Read the model definition and answer for the solid it produces. Units are mm, in the model's axes. A direction names the side the tool comes from. Round coordinates to 2 decimals unless told otherwise and drop trailing zeros. Write each loop counter-clockwise with the first axis right and the second up, starting at its lowest first coordinate (ties: lowest second). Pieces come first, ordered by that corner, then holes. Notation, with made-up numbers: (13.5, 15) - (43.5, 15) arc R4 cw to (43.5, 22) - close; hole circle Ø2 at (45, 7). An arc over 180 degrees is marked (long way). One line per item, written item: value. Start each with the question number.
(1) A cutting plane is placed at D-D, the plane x = 17. Determine the outline of the cut face in (y, z).
(2) Find the intervals of material crossed by L1, parallel to Y at x = 10, z = 24; L2, parallel to X at y = 21.5, z = 22; L3, parallel to Y at x = -71, z = 9.5, in increasing order.
(3) Flat-ended cylindrical pins translate along their axes: pin 1 Ø12 at (x, z) = (35, 26.5) entering from +Y; pin 2 Ø1 at (y, z) = (-17, 23.5) entering from +X; pin 3 Ø10 at (x, z) = (-56, 17.5) entering from -Y. Find the tip coordinate at first contact, or state that the pin passes through.
(4) A cutting plane is placed at B-B, the plane z = 20. Determine the outline of the cut face in (x, y).
(5) For faces 3 (the face through (0, 22.5, 14)), 4 (the face through (-62.735, 49.663, 15.818)), determine the directions among +Z, -Z, +X, -X, +Y, -Y from which every point of the face is accessible in a straight line to the end or side of a thin tool.
(6) The mould has two halves that part along Y. Classify faces 1 (the face through (-1, 28, 0)), 2 (the face through (63.45, -46.67, 29.16)): +Y half, -Y half, draft (parallel to the pull), parting line (faces both ways), or undercut.
(7) A cutting plane is placed at C-C, the plane y = 38. State how many separate pieces and enclosed holes the cut face has, plus the area to 3 significant figures.
(8) A cutting plane is placed at A-A, the plane x = -50. Determine the outline of the cut face in (y, z), plus the area to 3 significant figures.
from build123d import *

# Parameters (mm, degrees)
F1_DEPTH = 3
F2_DEPTH = 30
F3_SIZE  = 1


with BuildPart() as f1:
    # F0 (on Top) → F1 (new body)
    with BuildSketch(Plane.XY):
        with BuildLine():
            Line((13.857919263, 32.5), (-13.857919263, 32.5))
            ThreePointArc((-13.857919263, 32.5), (-66.5376476243, 56.1564438266), (-80, 0))
            ThreePointArc((-80, 0), (-66.5376476243, -56.1564438266), (-13.857919263, -32.5))
            Line((-13.857919263, -32.5), (13.857919263, -32.5))
            ThreePointArc((13.857919263, -32.5), (66.5376476243, -56.1564438266), (80, 0))
            ThreePointArc((80, 0), (66.5376476243, 56.1564438266), (13.857919263, 32.5))
        make_face()
        with BuildLine():
            ThreePointArc((-69.843134833, 0), (-63.4726862442, 49.30460269), (-20.1043481422, 25))
            Line((-20.1043481422, 25), (20.1043481422, 25))
            ThreePointArc((20.1043481422, 25), (63.4726862442, 49.30460269), (69.843134833, 0))
            ThreePointArc((69.843134833, 0), (63.4726862442, -49.30460269), (20.1043481422, -25))
            Line((20.1043481422, -25), (-20.1043481422, -25))
            ThreePointArc((-20.1043481422, -25), (-63.4726862442, -49.30460269), (-69.843134833, 0))
        make_face(mode=Mode.SUBTRACT)
    extrude(amount=F1_DEPTH)

    # F0 (on Top) → F2 (join)
    with BuildSketch(Plane.XY):
        with BuildLine():
            Line((20.1043481422, 25), (-20.1043481422, 25))
            ThreePointArc((-20.1043481422, 25), (-63.4726862442, 49.30460269), (-69.843134833, 0))
            ThreePointArc((-69.843134833, 0), (-63.4726862442, -49.30460269), (-20.1043481422, -25))
            Line((-20.1043481422, -25), (20.1043481422, -25))
            ThreePointArc((20.1043481422, -25), (63.4726862442, -49.30460269), (69.843134833, 0))
            ThreePointArc((69.843134833, 0), (63.4726862442, 49.30460269), (20.1043481422, 25))
        make_face()
        with BuildLine():
            ThreePointArc((-22.5, -22.5), (-62.677476518, -46.9035159175), (-65.8113883008, 0))
            ThreePointArc((-65.8113883008, 0), (-62.677476518, 46.9035159175), (-22.5, 22.5))
            Line((-22.5, 22.5), (22.5, 22.5))
            ThreePointArc((22.5, 22.5), (62.677476518, 46.9035159175), (65.8113883008, 0))
            ThreePointArc((65.8113883008, 0), (62.677476518, -46.9035159175), (22.5, -22.5))
            Line((22.5, -22.5), (-22.5, -22.5))
        make_face(mode=Mode.SUBTRACT)
    extrude(amount=F2_DEPTH)

    # F3
    f3_edges = [f1.edges().sort_by_distance(p)[0] for p in [
        (-63.472686, -49.304603, 30),
        (0, -25, 30),
        (63.472686, -49.304603, 30),
        (63.472686, 49.304603, 30),
        (0, 25, 30),
        (-63.472686, 49.304603, 30),
        (-62.677477, 46.903516, 30),
        (-62.677477, -46.903516, 30),
        (0, -22.5, 30),
        (0, 22.5, 30),
        (62.677477, 46.903516, 30),
        (62.677477, -46.903516, 30),
    ]]
    chamfer(f3_edges, length=F3_SIZE)


solid = f1.part
Here are the results:
1. outline: (-40.31, 0) - (-22.5, 0) - (-22.5, 29) - (-23.5, 30) - (-24, 30) - (-25, 29) - (-25, 3) - (-40.31, 3) - close; (22.5, 0) - (40.31, 0) - (40.31, 3) - (25, 3) - (25, 29) - (24, 30) - (23.5, 30) - (22.5, 29) - close
2. L1: -25 to -22.5, 22.5 to 25
2. L2: -79.98 to -77.48, 77.48 to 79.98
2. L3: -43.92 to -40.26, -4.74 to -1.08, 1.08 to 4.74, 40.26 to 43.92
3. pin 1: y = 51.12
3. pin 2: x = 79.58
3. pin 3: y = -52.48
4. outline: (-69.84, 0) arc R30 ccw (long way) to (-20.1, -25) - (20.1, -25) arc R30 ccw (long way) to (69.84, 0) arc R30 ccw (long way) to (20.1, 25) - (-20.1, 25) arc R30 ccw (long way) to start; hole (-65.81, 0) arc R27.5 ccw (long way) to (-22.5, -22.5) - (22.5, -22.5) arc R27.5 ccw (long way) to (65.81, 0) arc R27.5 ccw (long way) to (22.5, 22.5) - (-22.5, 22.5) arc R27.5 ccw (long way) to start
5. face 3: +Z, -Z
5. face 4: +Z
6. face 1: draft
6. face 2: undercut
7. separate pieces: 4
7. enclosed holes: 0
7. area: 453 mm²
8. outline: (-60, 0) - (-50, 0) - (-50, 29) - (-51, 30) - (-51.5, 30) - (-52.5, 29) - (-52.5, 3) - (-60, 3) - close; (50, 0) - (60, 0) - (60, 3) - (52.5, 3) - (52.5, 29) - (51.5, 30) - (51, 30) - (50, 29) - close
8. area: 193 mm²
